The model under review builds one solid part; all positions refer to its coordinate system, in mm. A direction names the side the tool comes from. Coordinates: 2 decimals unless noted, no trailing zeros. Order: outer loops, then holes, each group sorted by start corner. A loop starts at its lowest first (then second) coordinate and runs counter-clockwise, first axis right, second up.
Autodesk Inventor part; units mm, degrees
ref_plane "YZ Plane" through (0, 0, 0) normal (1, 0, 0) x (0, 1, 0)
ref_plane "XZ Plane" through (0, 0, 0) normal (0, 1, 0) x (-1, 0, 0)
ref_plane "XY Plane" through (0, 0, 0) normal (0, 0, 1) x (1, 0, 0)
sketch "Sketch1" plane through (0, 0, 0) normal (0, 0, 1) x (1, 0, 0)
  line L0 (0, 0) -> (-4, 0)
  line L1 (-4, 0) -> (-4, -14.15)
  line L2 (-4, -14.15) -> (0, -14.15)
  line L3 (0, -14.15) -> (0, 0)
  line L4 (0, 2.83) -> (0, -16.98)
  line L5 (-4.8, 0) -> (0.8, 0)
  dimension "d1" = 14.15
  dimension "d2" = 4
revolve "Shoulder" add sketch "Sketch1" angle 360 about axis through (0, -14.15, 0) along (0, 1, 0)
sketch "Sketch2" plane through (0, 0, 0) normal (0, 1, 0) x (1, 0, 0)
  circle A0 centre (0, 0) radius 4
  circle A1 centre (0, 0) radius 3.76
  dimension "d3" = 7.52
extrude "Shoulder_neck" add sketch "Sketch2" along normal blind 1.85 contours A1
sketch "Sketch3" plane through (0, 1.85, 0) normal (0, 1, 0) x (1, 0, 0)
  circle A0 centre (0, 0) radius 3.76
  circle A1 centre (0, 0) radius 6.6
  dimension "d6" = 13.2
extrude "Head" add sketch "Sketch3" along normal blind 5.5 contours A0 | A1
sketch "Sketch4" plane through (0, -14.15, 0) normal (0, -1, 0) x (1, 0, 0)
  circle A0 centre (0, 0) radius 4
  circle A1 centre (0, 0) radius 2.255
  dimension "d9" = 4.51
extrude "Thread_neck" add sketch "Sketch4" along normal blind 2.3 contours A1
sketch "Sketch5" plane through (0, -16.45, 0) normal (0, -1, 0) x (1, 0, 0)
  circle A0 centre (0, 0) radius 2.255
  circle A1 centre (0, 0) radius 3
  dimension "d12" = 6
extrude "Thread_shoulder" add sketch "Sketch5" along normal blind 8.7 contours A0 | A1
sketch "Sketch6" plane through (0, 7.35, 0) normal (0, 1, 0) x (1, 0, 0)
  circle A0 centre (0, 0) radius 6.6
  circle A1 centre (0, 0) radius 2 construction
  line L0 (-2, 1.1547) -> (-2, -1.1547)
  line L1 (-2, -1.1547) -> (0, -2.3094)
  line L2 (0, -2.3094) -> (2, -1.1547)
  line L3 (2, -1.1547) -> (2, 1.1547)
  line L4 (2, 1.1547) -> (0, 2.3094)
  line L5 (0, 2.3094) -> (-2, 1.1547)
  dimension "d15" = 4
extrude "Hex" cut sketch "Sketch6" against normal blind 3.3 contours L5 L4 L3 L2 L1 L0
chamfer "Chamfer1" distance 0.24 angle 30 1 edges at (4, 0, 0) measured on face at (-3.8448, 0, -0.619)
fillet "Fillet1" radius 0.4 1 edges at (-3.76, 1.85, 0)
chamfer "Chamfer2" distance 0.4 angle 30 1 edges at (-6.6, 7.35, 0) measured on face at (6.5145, 5.5167, 1.0587)
chamfer "Chamfer3" distance 0.5 angle 30 1 edges at (-3, -25.15, 0) measured on face at (0.929, -25.15, 0.823)
fillet "Fillet2" radius 0.6 1 edges at (-2.255, -14.15, 0)
chamfer "Chamfer7" distance 0.745 angle 30 1 edges at (-3, -16.45, 0) measured on face at (2.7008, -16.45, -0.4192)
thread "Thread"
equation "\"d2\" = 0.5 * Shoulder_diameter"
equation "\"d3\" = Shoulder_neck_dia"
equation "\"d4\" = Shoulder_neck_length"
equation "\"d6\" = Head_diameter"
equation "\"d7\" = Head_height"
equation "\"d9\" = Thread_neck_dia"
equation "\"d10\" = Thread_neck_length"
equation "\"d12\" = Thread_diameter"
equation "\"d13\" = Thread_length - Thread_neck_length"
equation "\"d15\" = Hex_size"
equation "\"d16\" = Hex_length"
equation "\"d18\" = -0.5 * Shoulder_neck_dia + 0.5 * Shoulder_diameter"
equation "\"d64\" = -0.5 * Shoulder_neck_dia + 0.5 * Shoulder_diameter"
equation "\"d21\" = 0.1 * Hex_size"
equation "\"d65\" = 0.1 * Hex_size"
equation "\"d23\" = 0.5 * Thread_pitch"
equation "\"d66\" = 0.5 * Thread_pitch"
equation "\"d25\" = Thread_neck_radius"
equation "\"d60\" = -0.5 * Thread_neck_dia + 0.5 * Thread_diameter"
equation "\"d67\" = -0.5 * Thread_neck_dia + 0.5 * Thread_diameter"
equation "\"Shoulder_diameter\" = 8"
equation "\"Shoulder_length\" = 35"
equation "\"Shoulder_neck_dia\" = 7.52"
equation "\"Thread_diameter\" = 6"
equation "\"Thread_length\" = 11"
equation "\"Head_diameter\" = 13.2"
equation "\"Head_height\" = 5.5"
equation "\"Thread_neck_dia\" = 4.51"
equation "\"Hex_size\" = 4"
equation "\"Hex_length\" = 3.3"
equation "\"Thread_pitch\" = 1"
equation "\"Shoulder_neck_length\" = 1.85"
equation "\"Thread_neck_length\" = 2.3"
equation "\"Thread_neck_radius\" = 0.6"
properties part number "SCREW, SHOULDER, P, 12.9,  M8X16MM" material "Steel, MS"
(1) Wall thickness on probe 1 along Y at (x, z) = (-6, 1); probe 2 along Z at (x, y) = (-1.5, 5.5); probe 3 along Y at (x, z) = (-1.75, -3): over which ranges is each line inside the solid? List them lowest first.
A:
probe 1: y = 1.85 to 7.35
probe 2: z = -6.43 to -1.44, 1.44 to 6.43
probe 3: y = -14.15 to 7.35
(2) For pin 1 Ø2 at (y, z) = (-14.5, -1) entering from +X; pin 2 Ø2 at (x, y) = (-2.5, -0.5) entering from +Z; pin 3 Ø2 at (x, y) = (-1, -10.5) entering from +Z, all flat-tipped, find the tip position at first contact; note any pin that passes through.
A:
pin 1: stops at x = 4
pin 2: stops at z = 3.71
pin 3: stops at z = 4
(3) We need section A-A, the plane y = 5. Write out the cut boundary in (x, z), and give its area (3 significant figures).
A:
outline: circle Ø13.2 at (0, 0); hole (-2, -1.15) - (0, -2.31) - (2, -1.15) - (2, 1.15) - (0, 2.31) - (-2, 1.15) - close
area: 123 mm2
(4) Machinability: for faces 1 (the face through (-2, 6, 0)), 2 (the face through (-2, 7.35, -2)), 3 (the face through (-3, -21, 0)), which of the approach directions +Z, -Z, +X, -X, +Y, -Y give a long, thin tool a straight path to every point of the face, cutting with its end or side? Answer none if there is none.
A:
face 1: +Y
face 2: +Z, -Z, +X, -X, +Y
face 3: -Y
(5) We need section C-C, the plane y = -10. Write out the cut boundary in (x, z).
A:
outline: circle Ø8 at (0, 0)
(6) Draft analysis for pull direction Y (two halves, no side actions). For faces 4 (the face through (3.586, 0.715, 1.129)), 5 (the face through (-1.014, 5.723, 1.724)), 6 (the face through (0, -25.15, 0)), 7 (the face through (0, 4.05, 0)), state which applies: released by +Y, released by -Y, zero draft, split by the parting line, or undercut.
A:
face 4: undercut
face 5: zero draft
face 6: released by -Y
face 7: released by +Y
(7) We need section B-B, the plane y = -19.5. Write out the cut boundary in (x, z).
A:
outline: circle Ø6 at (0, 0)
